Build history of the part. All positions in model axes, mm. Coordinates: 2 decimals unless noted, no trailing zeros. Loops run counter-clockwise (first coordinate to the right, second up) from the corner with the lowest first, then second, coordinate; pieces in that order, holes last. Notation, with made-up numbers: (21.5, 12.25) - (73.5, 12.25) arc R11 ccw to (73.5, 28.25) - close; hole circle Ø1 at (35.25, -27). An arc over 180 degrees is marked (long way). One line per item, written item: value.
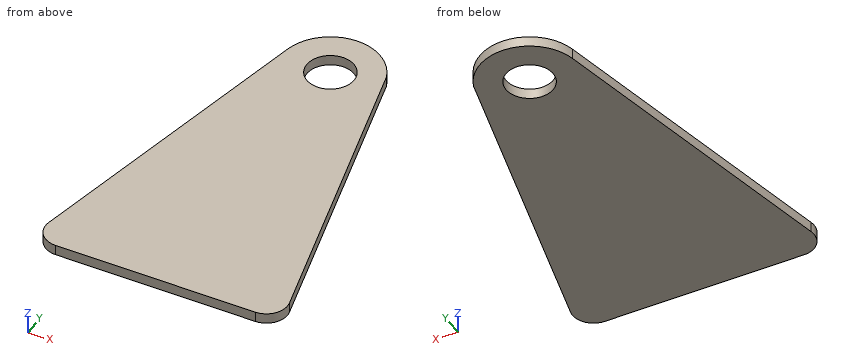
```python
from build123d import *

# Parameters (mm, degrees)
F0_R     = 14.2875
F1_DEPTH = 6.35


with BuildPart() as f1:
    # F0 (on Top) → F1 (new body)
    with BuildSketch(Plane.XY):
        with BuildLine():
            ThreePointArc((-72.658973, -75.862842), (-70.205698, -86.606139), (-60.276993, -91.387123))
            Line((-60.276993, -91.387123), (60.254503, -91.387123))
            ThreePointArc((60.254503, -91.387123), (70.188653, -86.599307), (72.632586, -75.845809))
            Line((72.632586, -75.845809), (28.183001, 117.79723))
            ThreePointArc((28.183001, 117.79723), (-2.110314, 137.138963), (-29.407204, 113.758043))
            Line((-29.407204, 113.758043), (-72.658973, -75.862842))
        make_face()
        with Locations((0, 107.050377)):
            Circle(F0_R, mode=Mode.SUBTRACT)
    extrude(amount=F1_DEPTH)


solid = f1.part
```
Item 1: Probe probe 1 along Y at (x, z) = (0, 2); probe 2 along Y at (x, z) = (7.5, 1); probe 3 along X at (y, z) = (117, 1.75). List the from-to ranges inside material, lowest first. Write a range as from..to.
Check result:
probe 1: y = -91.39..92.76, 121.34..137.21
probe 2: y = -91.39..94.89, 119.21..136.27
probe 3: x = -28.47..-10.25, 10.25..28.37
Item 2: Cut at D-D, the plane x = -17. Write the cut outline in (y, z), then the cut area to 3 significant figures.
Check result:
outline: (-91.39, 0) - (131.97, 0) - (131.97, 6.35) - (-91.39, 6.35) - close
area: 1,420 mm^2
Item 3: Cut at B-B, the plane z = 1.25. Write the cut outline in (x, y) (1 decimal).
Check result:
outline: (-72.7, -75.9) arc R12.7 ccw to (-60.3, -91.4) - (60.3, -91.4) arc R12.7 ccw to (72.6, -75.8) - (28.2, 117.8) arc R30.2 ccw to (-29.4, 113.8) - close; hole circle Ø28.6 at (0, 107.1)
Item 4: Drop flat-ended pins along their axis: P1, Ø2, axis at y = 35.5, z = 4.5, coming from the +X side; P2, Ø1.5, axis at x = 20.5, z = 2, coming from the +Y side. Give the stop position or say it passes through.
Check result:
P1: stops at x = 47.3
P2: stops at y = 129.85
Item 5: Cut at C-C, the plane y = -3. Write the cut outline in (x, z), then the cut area to 3 significant figures.
Check result:
outline: (-56.04, 0) - (55.91, 0) - (55.91, 6.35) - (-56.04, 6.35) - close
area: 711 mm^2
Item 6: Cut at A-A, the plane x = 0. Write the cut outline in (y, z).
Check result:
outline: (-91.39, 0) - (92.76, 0) - (92.76, 6.35) - (-91.39, 6.35) - close; (121.34, 0) - (137.21, 0) - (137.21, 6.35) - (121.34, 6.35) - close
